```python
from build123d import *

# Parameters (mm, degrees)
F0_R     = 9.525
F1_DEPTH = 3.175
F3_DEPTH = 1.524
F4_R     = 1.27
F5_DEPTH = 25.4
F6_R     = 2.3495
F7_DEPTH = 0.889


with BuildPart() as f1:
    # F0 (on Top) → F1 (new body)
    with BuildSketch(Plane.XY):
        Circle(F0_R)
    extrude(amount=F1_DEPTH)

    # F2 (on face) → F3 (cut)
    with BuildSketch(Plane.XY.offset(3.175)):
        with BuildLine():
            Line((2.3009442084, -2.794), (14.0832249425, -2.159))
            ThreePointArc((14.0832249425, -2.159), (16.129, 0), (14.0832249425, 2.159))
            Line((14.0832249425, 2.159), (2.3009442084, 2.794))
            ThreePointArc((2.3009442084, 2.794), (0, 3.6195), (-2.3009442084, 2.794))
            Line((-2.3009442084, 2.794), (-14.0832249425, 2.159))
            ThreePointArc((-14.0832249425, 2.159), (-16.129, 0), (-14.0832249425, -2.159))
            Line((-14.0832249425, -2.159), (-2.3009442084, -2.794))
            ThreePointArc((-2.3009442084, -2.794), (0, -3.6195), (2.3009442084, -2.794))
        make_face()
    extrude(amount=-F3_DEPTH, mode=Mode.SUBTRACT)

    # F4 (on face) → F5 (cut)
    with BuildSketch(Plane.XY.offset(1.651)):
        Circle(F4_R)
    extrude(amount=-F5_DEPTH, mode=Mode.SUBTRACT)

    # F6 (on face) → F7 (cut, through all)
    with BuildSketch(Plane(origin=(0, 0, 0), x_dir=(1, 0, 0), z_dir=(0, 0, -1))):
        Circle(F6_R)
    extrude(amount=-F7_DEPTH, mode=Mode.SUBTRACT)


solid = f1.part
```
Verification items for the finished model (mm, model axes). A direction names the side the tool comes from. Round coordinates to 2 decimals unless told otherwise and drop trailing zeros. Loops run counter-clockwise (first coordinate to the right, second up) from the corner with the lowest first, then second, coordinate; pieces in that order, holes last. Notation, with made-up numbers: (79.25, 88.5) -> (131.25, 88.5) arc R30 ccw to (131.25, 110.5) -> close; hole circle Ø4 at (65, 89.25). An arc over 180 degrees is marked (long way). Answer as a JSON object with one key per item and string values.
Q1. Draft check along X on faces 4 (the flat face through (0, 5, 3.175)), 5 (the cylindrical face through (-0.03, -3.62, 2.42)), 6 (the cylindrical face through (9.085, 2.861, 1.565)). Enter one of: pulls with the +X half, pulls with the -X half, needs draft (parallel to the pull), parting line crosses it, or undercut.
Data:
{"face 4": "needs draft", "face 5": "undercut", "face 6": "parting line crosses it"}
Q2. Scan lines: line 1 (Y direction, x = 0, z = 1.55) (3 decimals); line 2 (Y direction, x = 0, z = 0.6) (1 decimal); line 3 (Z direction, x = 2, y = 1.75). Record each from-to range of solid material in increasing order. Write a range as from..to.
Data:
{"line 1": "y = -9.525..-1.27, 1.27..9.525", "line 2": "y = -9.5..-2.3, 2.3..9.5", "line 3": "z = 0..1.65"}
Q3. Access from +Z, -Z, +X, -X, +Y, -Y to the whole of each face (thin tool, end or side, straight path). Record for faces 1 (the flat face through (2, -2, 0)), 2 (the cylindrical face through (-0.31, -2.33, 0.44)), 3 (the cylindrical face through (0.03, 3.62, 2.42)).
Data:
{"face 1": "-Z, +X, -X, +Y, -Y", "face 2": "-Z", "face 3": "+Z"}
Q4. Go/stop test with flat-tipped pins: P1, Ø1, axis at x = -1, z = 1.5, coming from the -Y side; P2, Ø1.4, axis at x = -0.5, y = 1, coming from the -Z side; P3, Ø3, axis at x = 0, y = 0, coming from the +Z side. Record where each tip stops, or that it passes through.
Data:
{"P1": "stops at y = -9.51", "P2": "stops at z = 0.89", "P3": "stops at z = 1.65"}
Q5. Section check B-B (x = 0). Record the boundary of the cut face in (y, z) (1 decimal), then the cut area to 3 significant figures.
Data:
{"outline": "(-9.5, 0) -> (-2.3, 0) -> (-2.3, 0.9) -> (-1.3, 0.9) -> (-1.3, 1.7) -> (-3.6, 1.7) -> (-3.6, 3.2) -> (-9.5, 3.2) -> close; (1.3, 0.9) -> (2.3, 0.9) -> (2.3, 0) -> (9.5, 0) -> (9.5, 3.2) -> (3.6, 3.2) -> (3.6, 1.7) -> (1.3, 1.7) -> close", "area": "43.3 mm2"}
Q6. Section check D-D (x = 8.25). Record the boundary of the cut face in (y, z) (3 decimals), then the cut area to 3 significant figures.
Data:
{"outline": "(-4.761, 0) -> (4.761, 0) -> (4.761, 3.175) -> (2.473, 3.175) -> (2.473, 1.651) -> (-2.473, 1.651) -> (-2.473, 3.175) -> (-4.761, 3.175) -> close", "area": "22.7 mm2"}
Q7. Section check A-A (y = 0). Record the boundary of the cut face in (x, z) (1 decimal).
Data:
{"outline": "(-9.5, 0) -> (-2.3, 0) -> (-2.3, 0.9) -> (-1.3, 0.9) -> (-1.3, 1.7) -> (-9.5, 1.7) -> close; (1.3, 0.9) -> (2.3, 0.9) -> (2.3, 0) -> (9.5, 0) -> (9.5, 1.7) -> (1.3, 1.7) -> close"}
